Autodesk Inventor part; units mm, degrees
ref_plane "YZ Plane" through (0, 0, 0) normal (1, 0, 0) x (0, 1, 0)
ref_plane "XZ Plane" through (0, 0, 0) normal (0, 1, 0) x (-1, 0, 0)
ref_plane "XY Plane" through (0, 0, 0) normal (0, 0, 1) x (1, 0, 0)
sketch "Эскиз3" plane through (0, 0, 0) normal (0, 1, 0) x (-1, 0, 0)
  circle A0 centre (0, 0) radius 5.5
  circle A1 centre (0, 0) radius 7.5
  line L0 (7.5, 0) -> (7.5, 7.5)
  line L1 (7.5, 7.5) -> (0, 7.5)
  line L2 (0, 7.5) -> (7.5, 7.5)
  line L3 (7.5, 7.5) -> (7.5, -7.5)
  line L4 (7.5, -7.5) -> (0, -7.5)
  line L5 (0, -7.5) -> (0, 7.5)
  line L6 (-7.5, 0) -> (-12.5, 0)
  circle A2 centre (-12.5, 0) radius 2.5
  circle A3 centre (-12.5, 0) radius 5
  line L7 (-1.5661, -7.3347) -> (-13.4999, -4.899)
  line L8 (-13.5, 4.899) -> (-1.5, 7.3485)
  line L9 (0, 5.5) -> (7.5, 5.5)
  line L10 (0, -5.5) -> (7.5, -5.5)
  line L11 (7.5, -5.5) -> (7.5, -4)
  line L12 (7.5, -4) -> (3.7749, -4)
  line L13 (7.5, 5.5) -> (7.5, 4)
  line L14 (7.5, 4) -> (3.7749, 4)
  circle A4 centre (0, 0) radius 2.45
  dimension "d9" = 11
  dimension "d10" = 15
  dimension "d11" = 5
  dimension "d12" = 5
  dimension "d13" = 1.5
  dimension "d14" = 1.5
  dimension "d17" = 4.9
extrude "Выдавливание3" add sketch "Эскиз3" along normal blind 4 contours A0 L14 A1 L12 | A0 L5 A1 | L5 A1 L9 | L14 L0 A1 | L10 A1 L5 | A1 L3 L12 | L1 L0 L9 A1 | A4 L5 | L5 A4 | A1 L10 L3 L4 | A1 A3 L8 | L7 A3 A1 | A2
sketch "Эскиз4" plane through (0, 4, 0) normal (0, 1, 0) x (1, 0, 0)
  circle A0 centre (12.5, 0) radius 2.5
  line L0 (1.5, -7.3485) -> (13.5, -4.899)
  circle A1 centre (12.5, 0) radius 5
  line L1 (-7.5, 7.5) -> (-7.5, 5.5)
  line L2 (-7.5, -7.5) -> (0, -7.5)
  line L3 (-7.5, 7.5) -> (-7.5, -7.5)
  line L4 (-7.5, -7.5) -> (0, -7.5)
  line L5 (1.5, -7.3485) -> (13.5, -4.899)
  arc A2 (1.5661, 7.3347) -> (0, 7.5) centre (0, 0) ccw
  line L6 (13.4999, 4.899) -> (1.5661, 7.3347)
  line L7 (1.5661, 7.3347) -> (13.4999, 4.899)
  line L8 (-7.5, 7.5) -> (0, 7.5)
  line L9 (0, 7.5) -> (-7.5, 7.5)
  circle A3 centre (0, 0) radius 7.5
  point P0 (0, 7.5)
extrude "Выдавливание4" add sketch "Эскиз4" along normal blind 2 contours A0 | A3 A1 L0 | A3 A2 | A1 | L2 L3 A3 | A3 L6 A1 | L3 L1 L8 A3
fillet "Сопряжение1" radius 1 2 edges at (13.5, 2, 4.899) (13.4999, 2, -4.899)
sketch "Эскиз5" plane through (0, 0, 0) normal (0, -1, 0) x (1, 0, 0)
  circle A0 centre (0, 0) radius 2.475
  circle A1 centre (12.5, 0) radius 2.5
  circle A2 centre (12.5, 0) radius 2.5
  dimension "d25" = 4.95
extrude "Выдавливание5" add sketch "Эскиз5" along normal blind 3 and the other way blind 5
fillet "Сопряжение3" radius 0.7 16 edges at (17.5, 6, -0.0001) (7.533, 6, -6.1168) (0.7538, 6, 7.462) (-3.75, 6, 7.5) (7.5, 6, 6.1237) (-7.5, 6, 0) (0.7874, 6, -7.4586) (-3.75, 6, -7.5) (-3.7749, 2, 4) (-3.7749, 2, -4) (-7.5, 2, -4) (-7.5, 2, -5.5) (-7.5, 4, -4.75) (-7.5, 2, 5.5) (-7.5, 2, 4) (-7.5, 4, 4.75)
properties part number "block_01"
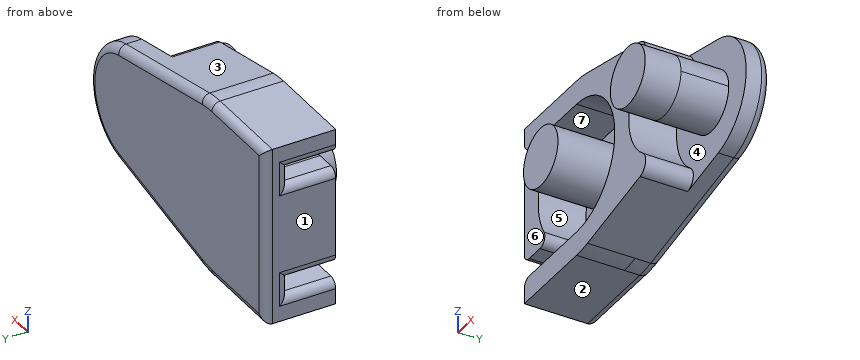
Can you work these out from the model? Positions are in its coordinate system, mm. Face numbers are marked on the shaded views. A direction names the side the tool comes from. Round coordinates to 2 decimals unless told otherwise and drop trailing zeros. Loops run counter-clockwise (first coordinate to the right, second up) from the corner with the lowest first, then second, coordinate; pieces in that order, holes last. Notation, with made-up numbers: (-38, 24.5) - (16, 24.5) arc R35 ccw to (16, 57.5) - close; hole circle Ø1 at (27, 13.5). An arc over 180 degrees is marked (long way). Answer in a Markdown table with one row per item. Add a question column.
Q1. I want a section at A-A on y = -1. List the corners of the cut face in (x, z) for me (3 decimals), and give its area (3 significant figures).
Q2. I need wall thicknesses on L1, parallel to Z at x = 0, y = 2.5 (3 decimals); L2, parallel to X at y = 1.75, z = 2; L3, parallel to Y at x = 16, z = 1. Which ranges of each line are inside material? Lowest first, please.
Q3. I want a section at B-B on x = -3.75. List the corners of the cut face in (y, z) for me, and give its area (3 significant figures).
Q4. I want a section at C-C on y = 1. Count the separate pieces of the cut face and the enclosed holes in it, and give its area (3 significant figures).
Q5. Which directions (+Z, -Z, +X, -X, +Y, -Y) give clear straight access to the entire face, cutting with the end or side of a thin tool? Please do the marked faces 5, 6 and 7.
Q6. We'd pull the mould along X, two halves only. Please class the marked faces 1, 2, 3 and 4: pulls with the +X half, pulls with the -X half, needs draft (parallel to the pull), parting line crosses it, or undercut.
Q7. For pin 1 Ø2 at (x, y) = (1.5, 4) entering from +Z; pin 2 Ø1.5 at (x, z) = (-6.5, 0) entering from -Y; pin 3 Ø4 at (x, y) = (10, 0) entering from +Z, each with a flat end and sliding along its axis, tell me the tip position at first contact or that it passes through.
A:
| question | item | result |
|---|---|---|
| 1 | outline | circle Ø4.95 at (0, 0); circle Ø5 at (12.5, 0) |
| 1 | area | 38.9 mm^2 |
| 2 | L1 | -7.5 to -5.5, -2.475 to 2.475, 5.5 to 7.5 |
| 2 | L2 | -7.5 to -5.12, -1.46 to 1.46, 5.12 to 7.92, 11 to 14 |
| 2 | L3 | 4 to 6 |
| 3 | outline | (0, -7.5) - (5.3, -7.5) arc R0.7 ccw to (6, -6.8) - (6, 6.8) arc R0.7 ccw to (5.3, 7.5) - (0, 7.5) - (0, 5.5) - (4, 5.5) - (4, -5.5) - (0, -5.5) - close |
| 3 | area | 45.8 mm^2 |
| 4 | separate pieces | 4 |
| 4 | enclosed holes | 0 |
| 4 | area | 157 mm^2 |
| 5 | face 5 | -Y |
| 5 | face 6 | +Z, -Z, -X, -Y |
| 5 | face 7 | -X, -Y |
| 6 | face 1 | pulls with the -X half |
| 6 | face 2 | needs draft |
| 6 | face 3 | pulls with the +X half |
| 6 | face 4 | undercut |
| 7 | pin 1 | z = 7.48 |
| 7 | pin 2 | y = 0 |
| 7 | pin 3 | z = 6.02 |
